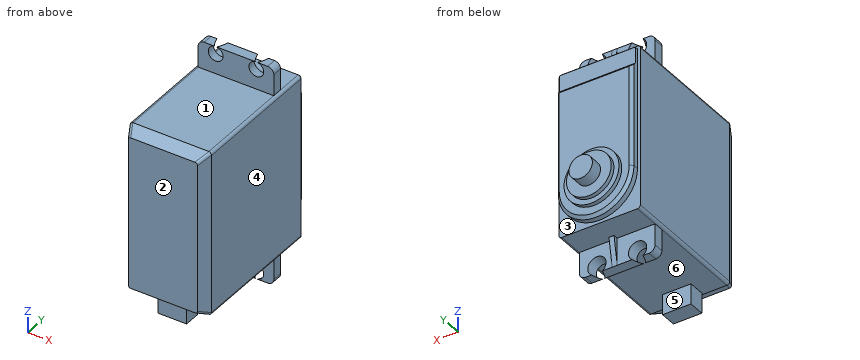
```python
from build123d import *

# Parameters (mm, degrees)
SKETCH1_W               = 20
SKETCH1_H               = 40.5
BOSS_EXTRUDE1_DEPTH     = 18
BOSS_EXTRUDE2_DEPTH     = 2
BOSS_EXTRUDE3_DEPTH     = 2.5
FILLET1_R               = 1.5
BOSS_EXTRUDE4_DEPTH     = 1.25
DRAFT1_ANGLE            = 10
SKETCH7_W               = 7
SKETCH7_H               = 4
BOSS_EXTRUDE5_DEPTH     = 5
CUT_EXTRUDE1_DEPTH      = 39.13135193
CUT_EXTRUDE1_DEPTH_BACK = 39.13135193
CHAMFER1_SIZE           = 0.7
CHAMFER2_SIZE           = 1.5
CHAMFER2_SIZE2          = 3
FILLET2_R               = 0.7


with BuildPart() as part:
    # Sketch1 → Boss-Extrude1 (new, symmetric)
    with BuildSketch(Plane(origin=(0, 0, 0), x_dir=(1, 0, 0), z_dir=(0, 1, 0))):
        Rectangle(SKETCH1_W, SKETCH1_H)
    extrude(amount=BOSS_EXTRUDE1_DEPTH, both=True)

    # Sketch2 → Boss-Extrude2 (add)
    with BuildSketch(Plane(origin=(0, 18, 0), x_dir=(1, 0, 0), z_dir=(0, 1, 0))):
        with BuildLine():
            Line((-9.3, 10.25), (-9.3, -19.55))
            Line((-9.3, -19.55), (9.3, -19.55))
            Line((9.3, -19.55), (9.3, 10.25))
            ThreePointArc((9.3, 10.25), (0, 19.55), (-9.3, 10.25))
        make_face()
    extrude(amount=BOSS_EXTRUDE2_DEPTH)

    # Sketch4 → Revolve1 (revolve)
    with BuildSketch(Plane(origin=(0, 0, 0), x_dir=(0, 0, -1), z_dir=(1, 0, 0))):
        Polygon((10.25, 20), (10.25, 25), (13.125, 25), (13.125, 22), (15.75, 22), (15.75, 21), (17, 21), (17, 20), align=None)
    revolve(axis=Axis((0, 20, -10.25), (0, 1, 0)))

    # Sketch5 → Boss-Extrude3 (add)
    with BuildSketch(Plane(origin=(0, 9, 0), x_dir=(-1, 0, 0), z_dir=(0, -1, 0))):
        with BuildLine():
            Line((-9.3, 20.25), (9.3, 20.25))
            Line((9.3, 20.25), (9.3, 27))
            Line((9.3, 27), (6.35, 27))
            ThreePointArc((6.35, 27), (5, 22.95), (3.65, 27))
            Line((3.65, 27), (-3.65, 27))
            ThreePointArc((-3.65, 27), (-5, 22.95), (-6.35, 27))
            Line((-6.35, 27), (-9.3, 27))
            Line((-9.3, 27), (-9.3, 20.25))
        make_face()
        with BuildLine():
            Line((9.3, -20.25), (-9.3, -20.25))
            Line((-9.3, -20.25), (-9.3, -27))
            Line((-9.3, -27), (-6.35, -27))
            ThreePointArc((-6.35, -27), (-5, -22.95), (-3.65, -27))
            Line((-3.65, -27), (3.65, -27))
            ThreePointArc((3.65, -27), (5, -22.95), (6.35, -27))
            Line((6.35, -27), (9.3, -27))
            Line((9.3, -27), (9.3, -20.25))
        make_face()
    extrude(amount=-BOSS_EXTRUDE3_DEPTH)

    # Fillet1
    fillet1_edges = [part.edges().sort_by_distance(p)[0] for p in [
        (-9.3, 10.25, -27),
        (9.3, 10.25, -27),
        (9.3, 10.25, 27),
        (-9.3, 10.25, 27),
    ]]
    fillet(fillet1_edges, radius=FILLET1_R)

    # Sketch6 → Boss-Extrude4 (add)
    with BuildSketch(Plane(origin=(0, 0, 0), x_dir=(0, 0, -1), z_dir=(1, 0, 0))):
        Polygon((20.25, 11.5), (27, 11.5), (20.25, 12.69020712), align=None)
        Polygon((-20.25, 12.69020712), (-20.25, 11.5), (-27, 11.5), align=None)
    extrude(amount=BOSS_EXTRUDE4_DEPTH)

    # Draft1
    draft1_faces = [part.faces().sort_by_distance(p)[0] for p in [
        (5, 10.25, 22.95),
        (-5, 10.25, 22.95),
        (-5, 10.25, -22.95),
        (5, 10.25, -22.95),
    ]]
    draft(draft1_faces, Plane.ZX.offset(11.5), DRAFT1_ANGLE)

    # Sketch7 → Boss-Extrude5 (add)
    with BuildSketch(Plane(origin=(0, 0, -20.25), x_dir=(-1, 0, 0), z_dir=(0, 0, -1))):
        with Locations((0, -12.5)):
            Rectangle(SKETCH7_W, SKETCH7_H)
    extrude(amount=BOSS_EXTRUDE5_DEPTH)

    # Sketch8 → Cut-Extrude1 (cut, two sides: drawn at the far end of the back side and taken through both)
    with BuildSketch(Plane(origin=(0, 0, 0), x_dir=(0, 0, -1), z_dir=(1, 0, 0)).offset(-CUT_EXTRUDE1_DEPTH_BACK)):
        Polygon((-19.55, 18.8), (-15.55, 18.8), (-14.35, 20), (-19.55, 20), align=None)
    extrude(amount=CUT_EXTRUDE1_DEPTH + CUT_EXTRUDE1_DEPTH_BACK, mode=Mode.SUBTRACT)

    # Chamfer1
    chamfer1_edges = [part.edges().sort_by_distance(p)[0] for p in [
        (9.3, 20, 2.05),
        (0, 20, -19.55),
        (-9.3, 20, 2.05),
    ]]
    chamfer(chamfer1_edges, length=CHAMFER1_SIZE)

    # Chamfer2
    chamfer2_edges = [part.edges().sort_by_distance(p)[0] for p in [
        (0, -18, 20.25),
        (-10, -18, 0),
        (0, -18, -20.25),
        (10, -18, 0),
    ]]
    chamfer2_side = [part.faces().sort_by_distance(p)[0] for p in [
        (0, -18, 0),
    ]]
    chamfer(chamfer2_edges, length=CHAMFER2_SIZE, length2=CHAMFER2_SIZE2, reference=chamfer2_side[0])

    # Fillet2
    # the kernel refuses this fillet: 0.7 mm, written as the material it takes off along each edge
    with BuildSketch(Plane(origin=(7.916666667, -19.166666667, 18.166666667), x_dir=(-0.9128709291752769, 0.365148371670112, 0.1825741858350529), z_dir=(0.4082482904638631, 0.8164965809277261, 0.4082482904638631)), Plane(origin=(7.916666667, -19.166666667, -18.166666667), x_dir=(0.18257418583505539, 0.36514837167011077, 0.9128709291752769), z_dir=(0.4082482904638631, 0.8164965809277261, -0.4082482904638631))) as fillet2_piece_1:
        with BuildLine():
            CenterArc((FILLET2_R * 0.816496580928, -FILLET2_R), FILLET2_R, 90, 78.463040967)
            Line((-FILLET2_R * 0.163299316186, -FILLET2_R * 0.8), (0, 0))
            Line((0, 0), (FILLET2_R * 0.816496580928, 0))
        make_face()
    extrude(amount=6.531972647, mode=Mode.SUBTRACT)
    with BuildSketch(Plane(origin=(-7.916666667, -19.166666667, 18.166666667), x_dir=(0.9128709291752769, 0.3651483716701107, 0.18257418583505536), z_dir=(-0.4082482904638631, 0.8164965809277261, 0.4082482904638631)), Plane(origin=(-7.916666667, -19.166666667, -18.166666667), x_dir=(-0.18257418583505539, 0.36514837167011077, 0.9128709291752769), z_dir=(-0.4082482904638631, 0.8164965809277261, -0.4082482904638631))) as fillet2_piece_2:
        with BuildLine():
            CenterArc((FILLET2_R * 0.816496580928, FILLET2_R), FILLET2_R, 191.536959033, 78.463040967)
            Line((-FILLET2_R * 0.163299316186, FILLET2_R * 0.8), (0, 0))
            Line((0, 0), (FILLET2_R * 0.816496580928, 0))
        make_face()
    extrude(amount=6.531972647, mode=Mode.SUBTRACT)
    with BuildSketch(Plane(origin=(10, -16.75, 20.25), x_dir=(-1, 0, 0), z_dir=(0, 1, 0)), Plane(origin=(-10, 19.75, 20.25), x_dir=(1, 0, 0), z_dir=(0, -1, 0)), Plane(origin=(-10, 19.75, -20.25), x_dir=(0, 0, 1), z_dir=(0, -1, 0)), Plane(origin=(10, -16.75, -20.25), x_dir=(0, 0, 1), z_dir=(0, 1, 0))) as fillet2_piece_3:
        with BuildLine():
            CenterArc((FILLET2_R, -FILLET2_R), FILLET2_R, 90, 90)
            Line((0, -FILLET2_R), (0, 0))
            Line((0, 0), (FILLET2_R, 0))
        make_face()
    extrude(amount=36.5, mode=Mode.SUBTRACT)


solid = part.part
```
Build history of the part. All positions in model axes, mm. Face numbers are marked on the shaded views. A direction names the side the tool comes from. Give positions to 0.01 mm unless a question says otherwise; leave off trailing zeros. Loops run counter-clockwise (first coordinate to the right, second up) from the corner with the lowest first, then second, coordinate; pieces in that order, holes last. Notation, with made-up numbers: (61, -6) -> (100, -6) arc R27 ccw to (100, 25) -> close; hole circle Ø10 at (-17, 78). An arc over 180 degrees is marked (long way). One line per question, with ' | ' between items. Start each with the question number.
1) Cut at C-C (z = 22). Give the cut face in (x, y).
2) Pin check, flat tips, straight feed: pin 1 (2 mm diameter, centred on x = 4, z = -23, fed in from +Y); pin 2 (1.2 mm diameter, centred on y = 11, z = -21.5, fed in from +X); pin 3 (3 mm diameter, centred on y = 10, z = 21.5, fed in from +X). Stop position of each tip, or through.
3) Cut at A-A (y = -6.5). Give the cut face in (x, z).
4) Two-plate mould, pull along Y, no slides. Class the marked faces 3, 4, 5 and 6: released by +Y, released by -Y, zero draft, split by the parting line, or undercut.
5) 3-axis set-ups, long thin cutter, end or side, ignore diameter. For the marked faces 1 and 2: which of +Z, -Z, +X, -X, +Y, -Y reach the whole face in a straight line?
6) Cut at B-B (z = 16.5). Give the cut face in (x, y).
7) Probe L1, parallel to Y at x = -2, z = -18; L2, parallel to Y at x = 6, z = -17.5; L3, parallel to Z at x = -1, y = 0. List the from-to ranges inside material, lowest first.
Return value:
1) outline: (-9.3, 9) -> (9.3, 9) -> (9.3, 11.5) -> (1.25, 11.5) -> (1.25, 12.38) -> (0, 12.38) -> (0, 11.5) -> (-9.3, 11.5) -> close
2) pin 1: y = 11.5 | pin 2: x = 9.3 | pin 3: x = 9.84
3) outline: (-10, -19.55) arc R0.7 ccw to (-9.3, -20.25) -> (9.3, -20.25) arc R0.7 ccw to (10, -19.55) -> (10, 19.55) arc R0.7 ccw to (9.3, 20.25) -> (-9.3, 20.25) arc R0.7 ccw to (-10, 19.55) -> close
4) face 3: released by +Y | face 4: zero draft | face 5: undercut | face 6: undercut
5) face 1: +Z, +X, -X, -Y | face 2: +Z, -Z, +X, -X, -Y
6) outline: (-10, -15) -> (-8.5, -18) -> (8.5, -18) -> (10, -15) -> (10, 18) -> (9.3, 18) -> (9.3, 18.8) -> (-9.3, 18.8) -> (-9.3, 18) -> (-10, 18) -> close
7) L1: -18 to 20 | L2: -18 to 18 | L3: -20.25 to 20.25
